Source: three-view drawing plus pictorial views. Frame: mm from the lowest corner of the part. A direction names the side the tool comes from. Give positions to 0.01 mm unless a question says otherwise; leave off trailing zeros. Write each loop counter-clockwise with the first axis right and the second up, starting at its lowest first coordinate (ties: lowest second). Pieces come first, ordered by that corner, then holes. Notation, with made-up numbers: (72.5, 71.5) -> (79.5, 71.5) arc R31 cw to (79.5, 105.5) -> close; hole circle Ø1 at (11.25, -17). An arc over 180 degrees is marked (long way). Write item = value, one per line.
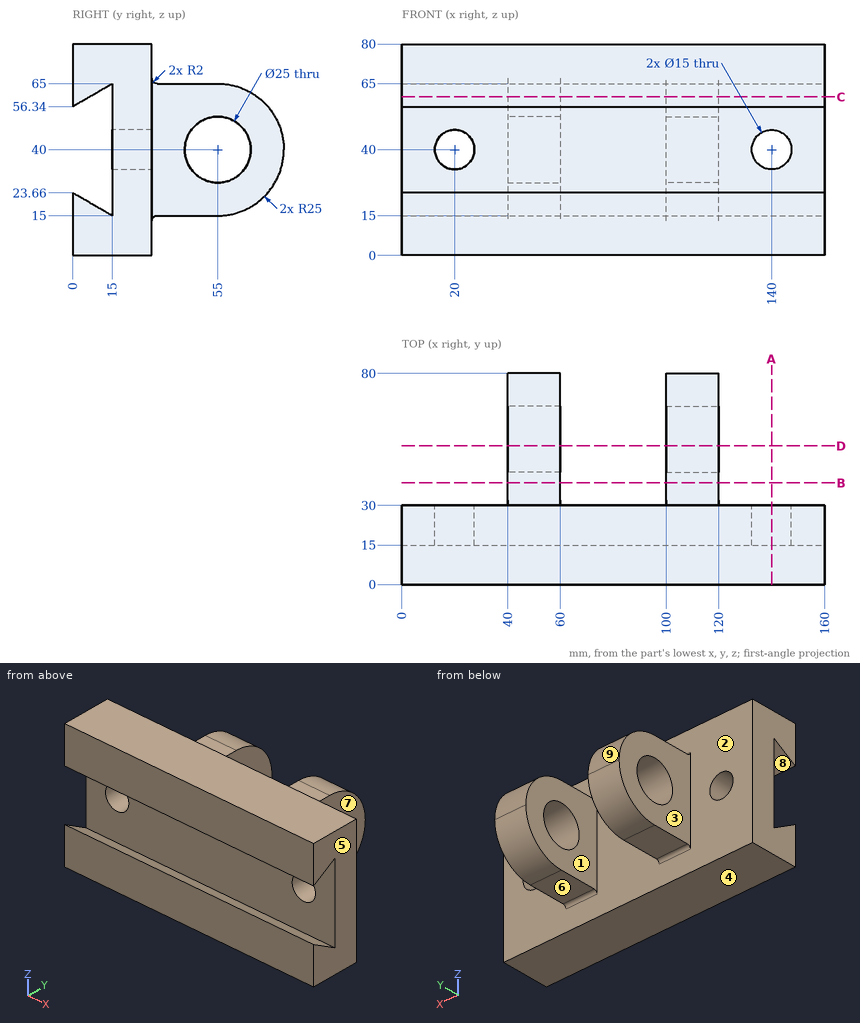
1) Cut plane A-A (x = 140). Return the cut outline in (y, z).
Computed:
outline = (0, 0) -> (30, 0) -> (30, 32.5) -> (15, 32.5) -> (15, 15) -> (0, 23.66) -> close; (0, 56.34) -> (15, 65) -> (15, 47.5) -> (30, 47.5) -> (30, 80) -> (0, 80) -> close
2) Contact query for flat-ended pins moving along their axis: pin 1 (10 mm diameter, centred on x = 47.5, y = 45.5, fed in from +Z); pin 2 (15 mm diameter, centred on y = 43.5, z = 35, fed in from +X); pin 3 (6 mm diameter, centred on x = 112.5, y = 38.5, fed in from -Z). Output: stop coordinate, or through.
Computed:
pin_1 = 65
pin_2 = 120
pin_3 = 15
3) Access query for the marked faces 5, 6, 7, 8 and 9. Directions: +Z, -Z, +X, -X, +Y, -Y. A direction counts if a zero-diameter tool reaches every point of the face in a straight line with its end or side. Return the directions, or none.
Computed:
face_5 = +Z, -Z, +X, +Y, -Y
face_6 = -Z, +X, -X, +Y
face_7 = +Z, -Z, +X, +Y
face_8 = +X, -X
face_9 = +Z, +X, -X, +Y
4) Cut plane C-C (z = 60). Return the cut outline in (x, y).
Computed:
outline = (0, 0) -> (160, 0) -> (160, 6.34) -> (0, 6.34) -> close; (0, 15) -> (160, 15) -> (160, 30) -> (120, 30) -> (120, 70) -> (100, 70) -> (100, 30) -> (60, 30) -> (60, 70) -> (40, 70) -> (40, 30) -> (0, 30) -> close
5) Material intervals for L1, parallel to X at y = 19, z = 40; L2, parallel to Y at x = 114.75, z = 40; L3, parallel to X at y = 67.5, z = 56, sorted ascending.
Computed:
L1 = 0 to 12.5, 27.5 to 132.5, 147.5 to 160
L2 = 15 to 42.5, 67.5 to 80
L3 = 40 to 60, 100 to 120
6) Draft query along X for the marked faces 1, 2, 3 and 4. Return one class per face: pulls with the +X half, pulls with the -X half, needs draft (parallel to the pull), parting line crosses it, or undercut.
Computed:
face_1 = undercut
face_2 = undercut
face_3 = pulls with the -X half
face_4 = needs draft
7) Cut plane D-D (y = 52.5). Return the cut outline in (x, z).
Computed:
outline = (40, 15) -> (60, 15) -> (60, 27.75) -> (40, 27.75) -> close; (40, 52.25) -> (60, 52.25) -> (60, 65) -> (40, 65) -> close; (100, 15) -> (120, 15) -> (120, 27.75) -> (100, 27.75) -> close; (100, 52.25) -> (120, 52.25) -> (120, 65) -> (100, 65) -> close
8) Cut plane B-B (y = 38.5). Return the cut outline in (x, z), then the cut area to 3 significant figures.
Computed:
outline = (40, 15) -> (60, 15) -> (60, 65) -> (40, 65) -> close; (100, 15) -> (120, 15) -> (120, 65) -> (100, 65) -> close
area = 2,000 mm²
